Input: part model. Units: mm. Frame: model coordinates. Give positions to 0.01 mm unless a question says otherwise; leave off trailing zeros. Loops run counter-clockwise (first coordinate to the right, second up) from the corner with the lowest first, then second, coordinate; pieces in that order, holes last. Notation, with made-up numbers: M 19,-39 L 65,-39 A9 cw 65,-31 Z; hole C -5.5,68 d5. An arc over 180 degrees is marked long. Return JSON: item names as keys, results as strings. Group by question number.
```python
from build123d import *

# Parameters (mm, degrees)
SKETCH1_W           = 9.652
SKETCH1_H           = 9.652
BOSS_EXTRUDE1_DEPTH = 33.02
SKETCH2_R           = 3.9878
CUT_EXTRUDE1_DEPTH  = 35.738620871


with BuildPart() as part:
    # Sketch1 → Boss-Extrude1 (new body)
    with BuildSketch(Plane(origin=(0, 0, 0), x_dir=(1, 0, 0), z_dir=(0, 1, 0))):
        Rectangle(SKETCH1_W, SKETCH1_H)
    extrude(amount=BOSS_EXTRUDE1_DEPTH)

    # Sketch2 → Cut-Extrude1 (cut, through all)
    with BuildSketch(Plane.XY.offset(4.826)):
        with Locations((0, 22.098)):
            Circle(SKETCH2_R)
        with Locations(Location((0, 10.922, 0), (0, 0, 180))):
            Circle(SKETCH2_R)
    extrude(amount=-CUT_EXTRUDE1_DEPTH, mode=Mode.SUBTRACT)


solid = part.part
```
Item 1: Material intervals for line 1 (Y direction, x = 0, z = 1); line 2 (X direction, y = 11, z = 2.75); line 3 (Y direction, x = -3, z = 2.5), sorted ascending. Write a range as from..to.
Item 2: Section B-B, the plane y = 23. Return loops of the section in (x, z), then the cut area to 3 significant figures.
Item 3: Section D-D, the plane x = -2.5. Return loops of the section in (y, z).
Item 4: Section A-A, the plane x = 0. Return loops of the section in (y, z), then the cut area to 3 significant figures.
Item 5: Section C-C, the plane z = -2. Return loops of the section in (x, y).
Item 6: Pull-direction query (Y, two-part tool) for faces 1 (the face through (-0.52, 26.05, 0.07)), 2 (the face through (0, 16, -4.826)), 3 (the face through (-2.144, 7.559, 0.068)), 4 (the face through (0, 0, 0)); classes: pulls with the +Y half, pulls with the -Y half, needs draft (parallel to the pull), parting line crosses it, or undercut.
Item 7: First-contact query: pin 1 Ø1 at (x, y) = (-3, 22.5) entering from +Z. Flat tip, straight axial feed; report the tip coordinate or a pass-through.
Answer below:
{
 "1": {"line 1": "0..6.93, 14.91..18.11, 26.09..33.02", "line 2": "-4.83..-3.99, 3.99..4.83", "line 3": "0..8.29, 13.55..19.47, 24.73..33.02"},
 "2": {"outline": "M -4.83,-4.83 L -3.88,-4.83 L -3.88,4.83 L -4.83,4.83 Z; M 3.88,-4.83 L 4.83,-4.83 L 4.83,4.83 L 3.88,4.83 Z", "area": "18.2 mm^2"},
 "3": {"outline": "M 0,-4.83 L 7.82,-4.83 L 7.82,4.83 L 0,4.83 Z; M 14.03,-4.83 L 18.99,-4.83 L 18.99,4.83 L 14.03,4.83 Z; M 25.2,-4.83 L 33.02,-4.83 L 33.02,4.83 L 25.2,4.83 Z"},
 "4": {"outline": "M 0,-4.83 L 6.93,-4.83 L 6.93,4.83 L 0,4.83 Z; M 14.91,-4.83 L 18.11,-4.83 L 18.11,4.83 L 14.91,4.83 Z; M 26.09,-4.83 L 33.02,-4.83 L 33.02,4.83 L 26.09,4.83 Z", "area": "165 mm^2"},
 "5": {"outline": "M -4.83,0 L 4.83,0 L 4.83,33.02 L -4.83,33.02 Z; hole C 0,10.92 d7.98; hole C 0,22.1 d7.98"},
 "6": {"face 1": "undercut", "face 2": "needs draft", "face 3": "undercut", "face 4": "pulls with the -Y half"},
 "7": {"pin 1": "through"}
}
